Geometry: see drawing. Coordinates: mm, zero at the bounding-box minimum. Round coordinates to 2 decimals unless told otherwise and drop trailing zeros. Write each loop counter-clockwise with the first axis right and the second up, starting at its lowest first coordinate (ties: lowest second). Pieces come first, ordered by that corner, then holes.
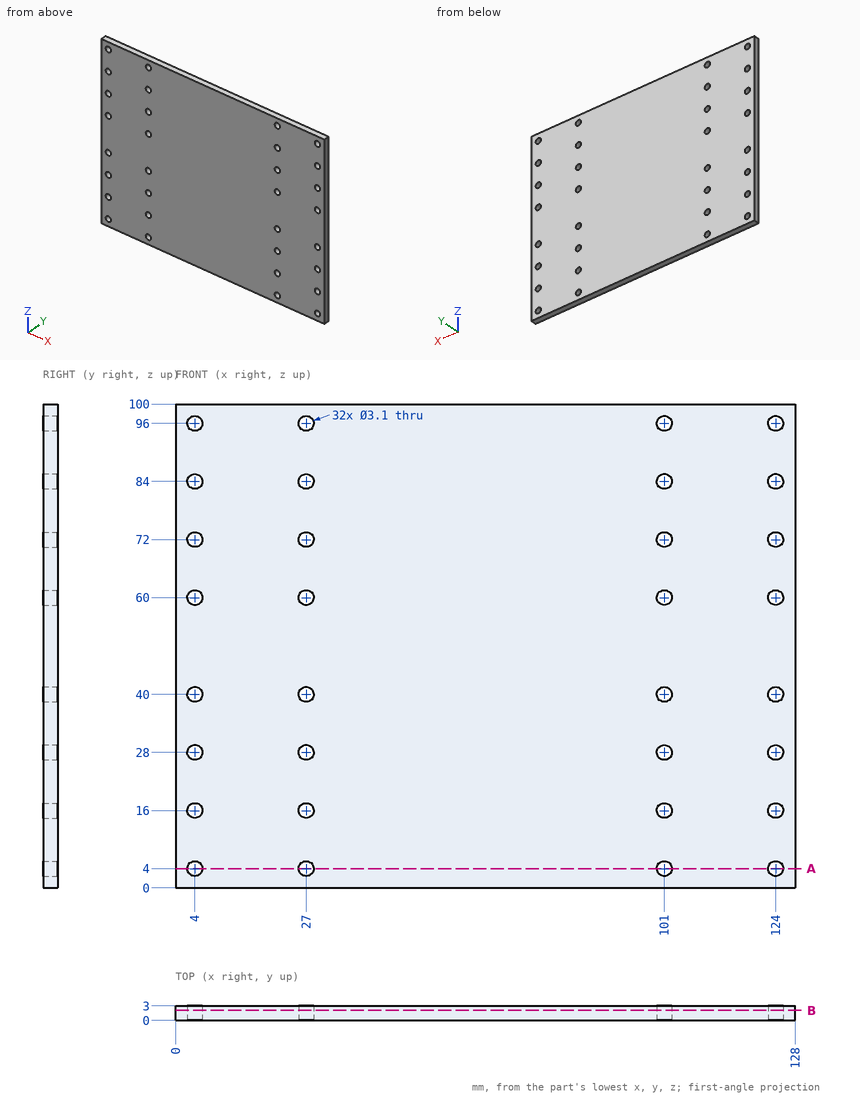
Q1. Section query A-A, the plane z = 4. Output: boundary loops of the cut face in (x, y), and give its area (3 significant figures).
Q2. Line query: line 1 (X direction, y = 1.2, z = 4); line 2 (X direction, y = 0.8, z = 59). Output: solid intervals per line, ascending.
Q3. Section query B-B, the plane y = 2.1. Give the number of separate pieces and of enclosed holes in the cut face, and give its area (3 significant figures).
Filled in:
1. outline: (0, 0) - (2.45, 0) - (2.45, 3) - (0, 3) - close; (5.55, 0) - (25.45, 0) - (25.45, 3) - (5.55, 3) - close; (28.55, 0) - (99.45, 0) - (99.45, 3) - (28.55, 3) - close; (102.55, 0) - (122.45, 0) - (122.45, 3) - (102.55, 3) - close; (125.55, 0) - (128, 0) - (128, 3) - (125.55, 3) - close
1. area: 347 mm2
2. line 1: x = 0 to 2.45, 5.55 to 25.45, 28.55 to 99.45, 102.55 to 122.45, 125.55 to 128
2. line 2: x = 0 to 2.82, 5.18 to 25.82, 28.18 to 99.82, 102.18 to 122.82, 125.18 to 128
3. separate pieces: 1
3. enclosed holes: 32
3. area: 12,600 mm2
